```python
from build123d import *

# Parameters (mm, degrees)
SKETCH1_W                      = 40
SKETCH1_H                      = 22
BOSS_EXTRUDE1_DEPTH            = 5
CBORE_FOR_M3_SHCS1_AT_2_COUNT  = 2
CBORE_FOR_M3_SHCS1_AT_2_PITCH  = 16
SKETCH6_W                      = 40
SKETCH6_H                      = 6
BOSS_EXTRUDE2_DEPTH            = 28.7
SKETCH7_W                      = 40
SKETCH7_H                      = 4.9
BOSS_EXTRUDE3_DEPTH            = 9.87
SKETCH8_W                      = 40
SKETCH8_H                      = 17.5
BOSS_EXTRUDE4_DEPTH            = 9.87
SKETCH18_W                     = 40
SKETCH18_H                     = 5
BOSS_EXTRUDE7_DEPTH            = 2
CBORE_FOR_M3_SHCS2_AT_2_COUNT  = 2
CBORE_FOR_M3_SHCS2_AT_2_PITCH  = 25.201777654
CHAMFER1_SIZE                  = 3
FILLET2_R                      = 1
M3_CLEARANCE_HOLE1_D           = 3.4
M3_CLEARANCE_HOLE1_CSINK_D     = 3.45
M3_CLEARANCE_HOLE1_CSINK_ANGLE = 90
FILLET3_R                      = 1
CUT_EXTRUDE1_DEPTH             = 3
BOSS_EXTRUDE6_START            = 5
BOSS_EXTRUDE6_DEPTH            = 5
BOSS_EXTRUDE8_START            = 3.5
SKETCH19_R                     = 3.275
SKETCH19_R_2                   = 3.25
SKETCH19_R_3                   = 1.725
BOSS_EXTRUDE8_DEPTH            = 3.5
BOSS_EXTRUDE9_START            = 2.5
SKETCH20_R                     = 3.25
SKETCH20_R_2                   = 1.7
BOSS_EXTRUDE9_DEPTH            = 2.5


with BuildPart() as part:
    # Sketch1 → Boss-Extrude1 (new body)
    with BuildSketch(Plane(origin=(0, 0, 0), x_dir=(1, 0, 0), z_dir=(0, 1, 0))):
        Rectangle(SKETCH1_W, SKETCH1_H)
    extrude(amount=BOSS_EXTRUDE1_DEPTH)

    # Sketch4 → CBORE for M3 SHCS1 (revolve, cut)
    with BuildSketch(Plane(origin=(8, 5, 7.5), x_dir=(0, 0, 1), z_dir=(1, 0, 0))):
        Polygon((0, 0), (0, 5), (1.7, 5), (1.7, 3), (3.25, 3), (3.25, 0.025), (3.275, 0), align=None)
    cbore_for_m3_shcs1 = revolve(axis=Axis((8, 11.35, 7.5), (0, -1, 0)), mode=Mode.SUBTRACT)

    # CBORE for M3 SHCS1 at 2: CBORE for M3 SHCS1 ×2
    with Locations(*[(-i * CBORE_FOR_M3_SHCS1_AT_2_PITCH, 0, 0) for i in range(1, CBORE_FOR_M3_SHCS1_AT_2_COUNT)]):
        add(cbore_for_m3_shcs1, mode=Mode.SUBTRACT)

    # Sketch6 → Boss-Extrude2 (add)
    with BuildSketch(Plane(origin=(0, 5, 0), x_dir=(1, 0, 0), z_dir=(0, 1, 0))):
        with Locations((0, 14)):
            Rectangle(SKETCH6_W, SKETCH6_H)
    extrude(amount=-BOSS_EXTRUDE2_DEPTH)

    # Sketch7 → Boss-Extrude3 (add)
    with BuildSketch(Plane(origin=(0, 0, -17), x_dir=(-1, 0, 0), z_dir=(0, 0, -1))):
        with Locations((0, -21.25)):
            Rectangle(SKETCH7_W, SKETCH7_H)
    extrude(amount=BOSS_EXTRUDE3_DEPTH)

    # Sketch8 → Boss-Extrude4 (add)
    with BuildSketch(Plane(origin=(0, 0, -17), x_dir=(-1, 0, 0), z_dir=(0, 0, -1))):
        with Locations((0, -3.75)):
            Rectangle(SKETCH8_W, SKETCH8_H)
    extrude(amount=BOSS_EXTRUDE4_DEPTH)

    # Sketch18 → Boss-Extrude7 (add)
    with BuildSketch(Plane.XY.offset(11)):
        with Locations((0, 2.5)):
            Rectangle(SKETCH18_W, SKETCH18_H)
    extrude(amount=BOSS_EXTRUDE7_DEPTH)

    # Sketch11 → CBORE for M3 SHCS2 (revolve, cut)
    with BuildSketch(Plane(origin=(-12.600888827, 5, -19.98), x_dir=(0, 0, 1), z_dir=(1, 0, 0))):
        Polygon((0, 0), (0, 28.7), (1.7, 28.7), (1.7, 3), (3.25, 3), (3.25, 0.025), (3.275, 0), align=None)
    cbore_for_m3_shcs2 = revolve(axis=Axis((-12.600888827, 11.35, -19.98), (0, -1, 0)), mode=Mode.SUBTRACT)

    # CBORE for M3 SHCS2 at 2: CBORE for M3 SHCS2 ×2
    with Locations(*[(i * CBORE_FOR_M3_SHCS2_AT_2_PITCH, 0, 0) for i in range(1, CBORE_FOR_M3_SHCS2_AT_2_COUNT)]):
        add(cbore_for_m3_shcs2, mode=Mode.SUBTRACT)

    # Chamfer1
    chamfer1_edges = [part.edges().sort_by_distance(p)[0] for p in [
        (0, -12.5, -26.87),
    ]]
    chamfer(chamfer1_edges, length=CHAMFER1_SIZE)

    # Fillet2
    fillet2_edges = [part.edges().sort_by_distance(p)[0] for p in [
        (20, -2.25, -26.87),
        (-20, -11.85, -11),
        (20, -11.85, -11),
        (20, -15.65, -17),
        (-20, -15.65, -17),
        (-20, -21.25, -26.87),
        (-20, -2.25, -26.87),
        (-20, 2.5, 13),
        (20, 2.5, 13),
    ]]
    fillet(fillet2_edges, radius=FILLET2_R)

    # M3 Clearance Hole1 (through all)
    with Locations(Plane(origin=(0, 5, 0), x_dir=(1, 0, 0), z_dir=(0, 1, 0))):
        with Locations((-8, 7.5), (8, 7.5)):
            CounterSinkHole(M3_CLEARANCE_HOLE1_D / 2, M3_CLEARANCE_HOLE1_CSINK_D / 2, counter_sink_angle=M3_CLEARANCE_HOLE1_CSINK_ANGLE)

    # Fillet3
    # the kernel refuses this fillet: 1 mm, written as the material it adds along each edge
    with BuildSketch(Plane(origin=(19, 0, -11), x_dir=(0, -1, 0), z_dir=(-1, 0, 0))) as fillet3_piece_1:
        with BuildLine():
            CenterArc((FILLET3_R, FILLET3_R), FILLET3_R, 180, 90)
            Line((0, FILLET3_R), (0, 0))
            Line((0, 0), (FILLET3_R, 0))
        make_face()
    extrude(amount=38)
    with BuildSketch(Plane(origin=(-19, 0, -12), x_dir=(0, 0, 1), z_dir=(1, 0, 0))) as fillet3_piece_2_section:
        with BuildLine():
            CenterArc((1 + FILLET3_R, FILLET3_R), FILLET3_R, 180, 90)
            Line((1 + FILLET3_R, 0), (1, 0))
            Line((1, 0), (1, FILLET3_R))
        make_face()
    fillet3_piece_2 = revolve(axis=Axis((-19, 0, -12), (0, -1, 0)), revolution_arc=233.296989237, mode=Mode.PRIVATE)
    fillet3_piece_2 = split(fillet3_piece_2, bisect_by=Plane(origin=(-20, -0.311628018, -11.250060985), z_dir=(1, 0, 0)), keep=Keep.TOP, mode=Mode.PRIVATE)
    add(fillet3_piece_2)
    with BuildSketch(Plane(origin=(19, 0, -12), x_dir=(-0.8017442392976477, 0, -0.5976672776328282), z_dir=(-0.5976672776328282, 0, 0.8017442392976477))) as fillet3_piece_3_section:
        with BuildLine():
            CenterArc((1 + FILLET3_R, FILLET3_R), FILLET3_R, 180, 90)
            Line((1, FILLET3_R), (1, 0))
            Line((1, 0), (1 + FILLET3_R, 0))
        make_face()
    fillet3_piece_3 = revolve(axis=Axis((19, 0, -12), (0, -1, 0)), revolution_arc=233.296989237, mode=Mode.PRIVATE)
    fillet3_piece_3 = split(fillet3_piece_3, bisect_by=Plane(origin=(20, -0.31162852, -11.250061149), z_dir=(-1, 0, 0)), keep=Keep.TOP, mode=Mode.PRIVATE)
    add(fillet3_piece_3)

    # Sketch15 → Cut-Extrude1 (cut)
    with BuildSketch(Plane.XZ.offset(23.7)):
        Polygon((15.900888827, -19.98), (14.250888827, -17.122116168), (10.950888827, -17.122116168), (9.300888827, -19.98), (10.950888827, -22.837883832), (14.250888827, -22.837883832), align=None)
        Polygon((-9.300888827, -19.98), (-10.950888827, -17.122116168), (-14.250888827, -17.122116168), (-15.900888827, -19.98), (-14.250888827, -22.837883832), (-10.950888827, -22.837883832), align=None)
    extrude(amount=-CUT_EXTRUDE1_DEPTH, mode=Mode.SUBTRACT)

    # Sketch16 → Boss-Extrude6 (add)
    with BuildSketch(Plane.XZ.offset(23.7).offset(BOSS_EXTRUDE6_START)):
        with BuildLine():
            Line((19, -11), (-19, -11))
            ThreePointArc((-19, -11), (-19.707106781, -11.292893219), (-20, -12))
            Line((-20, -12), (-20, -25.87))
            ThreePointArc((-20, -25.87), (-19.707106781, -26.577106781), (-19, -26.87))
            Line((-19, -26.87), (20, -26.87))
            Line((20, -26.87), (20, -12))
            ThreePointArc((20, -12), (19.707106781, -11.292893219), (19, -11))
        make_face()
        Polygon((10.950888827, -22.837883832), (14.250888827, -22.837883832), (15.900888827, -19.98), (14.250888827, -17.122116168), (10.950888827, -17.122116168), (9.300888827, -19.98), align=None, mode=Mode.SUBTRACT)
        Polygon((-10.950888827, -22.837883832), (-9.300888827, -19.98), (-10.950888827, -17.122116168), (-14.250888827, -17.122116168), (-15.900888827, -19.98), (-14.250888827, -22.837883832), align=None, mode=Mode.SUBTRACT)
    extrude(amount=-BOSS_EXTRUDE6_DEPTH)

    # Sketch19 → Boss-Extrude8 (add)
    with BuildSketch(Plane(origin=(0, 5, 0), x_dir=(1, 0, 0), z_dir=(0, 1, 0)).offset(BOSS_EXTRUDE8_START)):
        with BuildLine():
            Line((-19, -13), (19, -13))
            ThreePointArc((19, -13), (19.707106781, -12.707106781), (20, -12))
            Line((20, -12), (20, 25.87))
            ThreePointArc((20, 25.87), (19.707106781, 26.577106781), (19, 26.87))
            Line((19, 26.87), (-19, 26.87))
            ThreePointArc((-19, 26.87), (-19.707106781, 26.577106781), (-20, 25.87))
            Line((-20, 25.87), (-20, -12))
            ThreePointArc((-20, -12), (-19.707106781, -12.707106781), (-19, -13))
        make_face()
        with Locations(Location((-8, -7.5, 0), (0, 0, 270))):
            Circle(SKETCH19_R, mode=Mode.SUBTRACT)
        with Locations(Location((8, -7.5, 0), (0, 0, 270))):
            Circle(SKETCH19_R_2, mode=Mode.SUBTRACT)
        with Locations(Location((8, 7.5, 0), (0, 0, 270))):
            Circle(SKETCH19_R_3, mode=Mode.SUBTRACT)
        with Locations(Location((-8, 7.5, 0), (0, 0, 270))):
            Circle(SKETCH19_R_3, mode=Mode.SUBTRACT)
        with Locations(Location((-12.600888827, 19.98, 0), (0, 0, 270))):
            Circle(SKETCH19_R_2, mode=Mode.SUBTRACT)
        with Locations(Location((12.600888827, 19.98, 0), (0, 0, 270))):
            Circle(SKETCH19_R, mode=Mode.SUBTRACT)
    extrude(amount=-BOSS_EXTRUDE8_DEPTH)

    # Sketch20 → Boss-Extrude9 (add)
    # profile 1 of 2: a face of its own
    with BuildSketch(Plane(origin=(0, 2, 0), x_dir=(1, 0, 0), z_dir=(0, 1, 0)).offset(BOSS_EXTRUDE9_START)):
        with Locations(Location((-8, -7.5, 0), (0, 0, 270))):
            Circle(SKETCH20_R)
        with Locations(Location((-8, -7.5, 0), (0, 0, 270))):
            Circle(SKETCH20_R_2, mode=Mode.SUBTRACT)
    # profile 2 of 2: a face of its own
    with BuildSketch(Plane(origin=(0, 2, 0), x_dir=(1, 0, 0), z_dir=(0, 1, 0)).offset(BOSS_EXTRUDE9_START)):
        with Locations(Location((8, -7.5, 0), (0, 0, 270))):
            Circle(SKETCH20_R)
        with Locations(Location((8, -7.5, 0), (0, 0, 270))):
            Circle(SKETCH20_R_2, mode=Mode.SUBTRACT)
    extrude(amount=-BOSS_EXTRUDE9_DEPTH)


solid = part.part
```
Geometry check sheet. Reference: the model listing, model coordinates, mm. A direction names the side the tool comes from. Give positions to 0.01 mm unless a question says otherwise; leave off trailing zeros. Write each loop counter-clockwise with the first axis right and the second up, starting at its lowest first coordinate (ties: lowest second). Pieces come first, ordered by that corner, then holes.
1) Gauge pin test, flat ends, axial feed: pin 1 (5 mm diameter, centred on x = -12.6, z = -19.98, fed in from +Y); pin 2 (5 mm diameter, centred on x = 8, z = 7.5, fed in from +Y); pin 3 (6.5 mm diameter, centred on x = 14, z = -19, fed in from -Y); pin 4 (3 mm diameter, centred on x = 13, y = -4, fed in from +Z). Record the tip position at first contact, or that the pin passes through.
2) Section check C-C, the plane y = -7.5. Record the boundary of the cut face in (x, z), and give its area (3 significant figures).
3) Section check A-A, the plane x = 8. State how many separate pieces and enclosed holes the cut face has, and give its area (3 significant figures).
4) Release check for a two-part mould opening along X. For faces 1 (the cylindrical face through (15.774, 3.508, -20.685)), 2 (the flat face through (0, 8.5, -7)) record: pulls with the +X half, pulls with the -X half, needs draft (parallel to the pull), parting line crosses it, or undercut.
5) Section check D-D, the plane z = 2. Record the boundary of the cut face in (x, y).
6) Material ranges on L1, parallel to Z at x = -8, y = 4.85; L2, parallel to X at y = 3.7, z = 7.5; L3, parallel to Y at x = -6.5, z = -23.5, recorded low to high.
7) Access from +Z, -Z, +X, -X, +Y, -Y to the whole of each face (thin tool, end or side, straight path). Record for faces 3 (the flat face through (0, -24, -26.87)), 4 (the cylindrical face through (10.197, 6.774, 5.105)), 5 (the cylindrical face through (-13.75, -19.737, -21.233)), 6 (the flat face through (0, -16, -17)), 7 (the flat face through (-13, -25, -22.838)).
Computed:
1. pin 1: stops at y = 2
1. pin 2: stops at y = 4.5
1. pin 3: stops at y = -28.7
1. pin 4: stops at z = -11
2. outline: (-20, -25.87) arc R1 ccw to (-19, -26.87) - (19, -26.87) arc R1 ccw to (20, -25.87) - (20, -12) arc R1 ccw to (19, -11) - (-19, -11) arc R1 ccw to (-20, -12) - close; hole circle Ø3.4 at (-12.6, -19.98); hole circle Ø3.4 at (12.6, -19.98)
2. area: 616 mm2
3. separate pieces: 3
3. enclosed holes: 0
3. area: 658 mm2
4. face 1: undercut
4. face 2: needs draft
5. outline: (-20, 0) - (20, 0) - (20, 8.5) - (-20, 8.5) - close
6. L1: z = -26.87 to -9.2, -5.8 to 4.25, 10.75 to 13
6. L2: x = -20 to -9.7, -6.3 to 6.3, 9.7 to 20
6. L3: y = -28.7 to -18.8, -12.5 to 8.5
7. face 3: -Z, +X, -X, +Y, -Y
7. face 4: +Y
7. face 5: +Y, -Y
7. face 6: -Z, +X, -X
7. face 7: -Y
